Model file for the job. Use its own axes, mm. Face numbers are marked on the shaded views. Round coordinates to 2 decimals unless told otherwise and drop trailing zeros. Order: outer loops, then holes, each group sorted by start corner. A loop starts at its lowest first (then second) coordinate and runs counter-clockwise, first axis right, second up. Notation, with made-up numbers: M 81.5,55 L 109.5,55 A20 ccw 109.5,79 Z; hole C 57.25,-38 d10. An arc over 180 degrees is marked long. Return JSON: item names as keys, results as strings. Group by question number.
Item 1: Pin check, flat tips, straight feed: pin 1 Ø4 at (x, z) = (-14, 19) entering from +Y; pin 2 Ø0.8 at (y, z) = (10.5, -2) entering from -X; pin 3 Ø1.5 at (x, z) = (-10.5, -2.5) entering from -Y; pin 4 Ø4 at (x, y) = (15, 3.5) entering from -Z. Stop position of each tip, or through.
Item 2: Slice it at B-B on z = 28.5. Write the cut outline in (x, y), then the cut area to 3 significant figures.
Item 3: Pull direction X, two halves, no side cores. Call the marked faces 1, 2 and 3: pulls with the +X half, pulls with the -X half, needs draft (parallel to the pull), parting line crosses it, or undercut.
Item 4: Slice it at A-A on x = -16.35. Write the cut outline in (y, z).
Item 5: Probe line 1 along Y through (x, z) = (-7, -8); line 2 along X through (y, z) = (5.25, 0.5); line 3 along Y through (x, z) = (14.5, -3.5). List the from-to ranges inside material, lowest first.
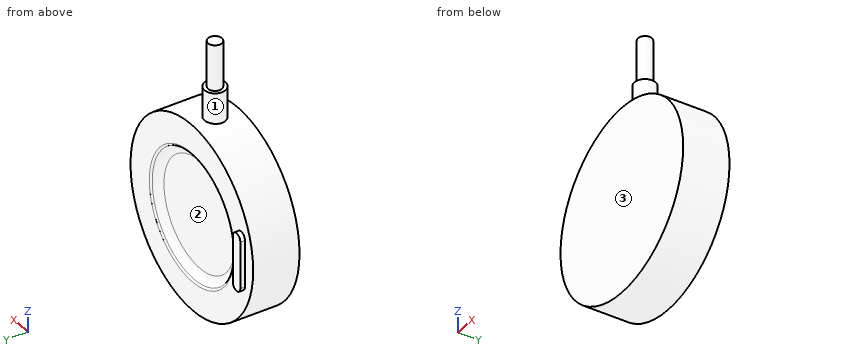
from build123d import *

# Parameters (mm, degrees)
SKETCH_1_R          = 20.3
EXTRUDE_1_DEPTH     = 10
SKETCH_2_R          = 2.3
EXTRUDE_2_DEPTH     = 26.9
SKETCH_3_R          = 1.5
EXTRUDE_3_DEPTH     = 10
EXTRUDE_4_DEPTH     = 1
SKETCH_5_R          = 13.7
CUT_EXTRUDE_1_DEPTH = 1.63
FILLET_1_R          = 2
FILLET_2_R          = 0.5


with BuildPart() as part:
    # 草图1 → 凸台-拉伸1 (new body)
    with BuildSketch(Plane(origin=(0, 0, 0), x_dir=(1, 0, 0), z_dir=(0, 1, 0))):
        with Locations(Location((0, 0, 0), (0, 0, 270))):
            Circle(SKETCH_1_R)
    extrude(amount=EXTRUDE_1_DEPTH)

    # 草图2 → 凸台-拉伸2 (add)
    with BuildSketch(Plane.XY):
        with Locations(Location((0, 5, 0), (0, 0, 180))):
            Circle(SKETCH_2_R)
    extrude(amount=EXTRUDE_2_DEPTH)

    # 草图3 → 凸台-拉伸3 (add)
    with BuildSketch(Plane.XY.offset(26.9)):
        with Locations((0, 5)):
            Circle(SKETCH_3_R)
    extrude(amount=EXTRUDE_3_DEPTH)

    # 草图4 → 凸台-拉伸4 (add)
    with BuildSketch(Plane(origin=(0, 10, 0), x_dir=(1, 0, 0), z_dir=(0, 1, 0))):
        with BuildLine():
            Line((-15.1, 5.1), (-15.1, -5.1))
            ThreePointArc((-15.1, -5.1), (-16.35, -6.35), (-17.6, -5.1))
            Line((-17.6, -5.1), (-17.6, 5.1))
            ThreePointArc((-17.6, 5.1), (-16.35, 6.35), (-15.1, 5.1))
        make_face()
    extrude(amount=EXTRUDE_4_DEPTH)

    # 草图5 → 切除-拉伸1 (cut)
    with BuildSketch(Plane(origin=(0, 10, 0), x_dir=(1, 0, 0), z_dir=(0, 1, 0))):
        with Locations(Location((0, 0, 0), (0, 0, 270))):
            Circle(SKETCH_5_R)
    extrude(amount=-CUT_EXTRUDE_1_DEPTH, mode=Mode.SUBTRACT)

    # 圆角1
    # the kernel refuses this fillet: 2 mm, written as the material it adds along each edge
    with BuildSketch(Plane(origin=(0, 8.37, 0), x_dir=(0, 0, 1), z_dir=(-1, 0, 0))) as fillet_1_piece_1:
        with BuildLine():
            CenterArc((11.734522959, 2), FILLET_1_R, 270, 79.338867602)
            Line((11.734522959, 0), (11.734522959, -0.04))
            Line((11.734522959, -0.04), (13.7, -0.04))
            Line((13.7, -0.04), (13.74, 0))
            ThreePointArc((13.74, 0), (13.74, 0.815), (13.739309541, 1.6226))
            Line((13.739309541, 1.6226), (13.7, 1.63))
        make_face()
    revolve(axis=Axis((0, 8.37, 0), (0, 1, 0)))

    # 圆角2
    fillet_2_edges = [part.edges().sort_by_distance(p)[0] for p in [
        (0, 10, -13.7),
    ]]
    fillet(fillet_2_edges, radius=FILLET_2_R)


solid = part.part
Output values:
{
 "1": {"pin 1": "through", "pin 2": "x = -17.6", "pin 3": "y = 0", "pin 4": "z = -15.59"},
 "2": {"outline": "C 0,5 d3", "area": "7.07 mm²"},
 "3": {"face 1": "parting line crosses it", "face 2": "undercut", "face 3": "needs draft"},
 "4": {"outline": "M 0,-12.03 L 10,-12.03 L 10,-6.35 L 11,-6.35 L 11,6.35 L 10,6.35 L 10,12.03 L 0,12.03 Z"},
 "5": {"line 1": "0 to 8.37", "line 2": "-20.29 to 20.29", "line 3": "0 to 10"}
}
